from build123d import *

# Parameters (mm, degrees)
F1_DEPTH = 15.875
F2_DEPTH = 3.3528
F3_DEPTH = 5.08
F4_R     = 5.08
F5_R     = 1.27


with BuildPart() as f1:
    # F0 (on Top) → F1 (new body)
    with BuildSketch(Plane.XY):
        Polygon((0, 25.4), (0, 0), (33.02, 0), (66.04, 0), (76.2, 0), (86.36, 0), (119.38, 0), (152.4, 0), (152.4, 33.02), (152.4, 68.58), (152.4, 101.6), (127, 101.6), (76.2, 101.6), (25.4, 101.6), (0, 101.6), (0, 76.2), align=None)
        with BuildLine():
            ThreePointArc((44.0314886751, 33.02), (45.151447055, 29.2829253769), (45.5295, 25.4))
            ThreePointArc((45.5295, 25.4), (8.6879749843, 14.179260714), (33.02, 44.0314886751))
            Line((33.02, 44.0314886751), (33.02, 57.5685113249))
            ThreePointArc((33.02, 57.5685113249), (8.6879749843, 87.420739286), (45.5295, 76.2))
            ThreePointArc((45.5295, 76.2), (45.151447055, 72.3170746231), (44.0314886751, 68.58))
            Line((44.0314886751, 68.58), (57.5685113249, 68.58))
            ThreePointArc((57.5685113249, 68.58), (72.3170746231, 95.951447055), (96.3295, 76.2))
            ThreePointArc((96.3295, 76.2), (95.951447055, 72.3170746231), (94.8314886751, 68.58))
            Line((94.8314886751, 68.58), (108.3685113249, 68.58))
            ThreePointArc((108.3685113249, 68.58), (123.1170746231, 95.951447055), (147.1295, 76.2))
            ThreePointArc((147.1295, 76.2), (138.220739286, 59.4879749843), (119.38, 57.5685113249))
            Line((119.38, 57.5685113249), (119.38, 44.0314886751))
            ThreePointArc((119.38, 44.0314886751), (138.220739286, 42.1120250157), (147.1295, 25.4))
            ThreePointArc((147.1295, 25.4), (123.1170746231, 5.648552945), (108.3685113249, 33.02))
            Line((108.3685113249, 33.02), (94.8314886751, 33.02))
            ThreePointArc((94.8314886751, 33.02), (95.951447055, 29.2829253769), (96.3295, 25.4))
            ThreePointArc((96.3295, 25.4), (72.3170746231, 5.648552945), (57.5685113249, 33.02))
            Line((57.5685113249, 33.02), (44.0314886751, 33.02))
        make_face(mode=Mode.SUBTRACT)
        with BuildLine():
            ThreePointArc((45.5295, 76.2), (8.6879749843, 87.420739286), (33.02, 57.5685113249))
            ThreePointArc((33.02, 57.5685113249), (39.6337059519, 61.9662940481), (44.0314886751, 68.58))
            ThreePointArc((44.0314886751, 68.58), (45.151447055, 72.3170746231), (45.5295, 76.2))
        make_face()
        with BuildLine():
            ThreePointArc((33.02, 44.0314886751), (8.6879749843, 14.179260714), (45.5295, 25.4))
            ThreePointArc((45.5295, 25.4), (45.151447055, 29.2829253769), (44.0314886751, 33.02))
            ThreePointArc((44.0314886751, 33.02), (39.6337059519, 39.6337059519), (33.02, 44.0314886751))
        make_face()
        with BuildLine():
            ThreePointArc((66.04, 42.7773176943), (61.0000405534, 38.5968936902), (57.5685113249, 33.02))
            ThreePointArc((57.5685113249, 33.02), (72.3170746231, 5.648552945), (96.3295, 25.4))
            ThreePointArc((96.3295, 25.4), (95.951447055, 29.2829253769), (94.8314886751, 33.02))
            ThreePointArc((94.8314886751, 33.02), (91.3999594466, 38.5968936902), (86.36, 42.7773176943))
            ThreePointArc((86.36, 42.7773176943), (76.2, 45.5295), (66.04, 42.7773176943))
        make_face()
        with BuildLine():
            ThreePointArc((147.1295, 76.2), (123.1170746231, 95.951447055), (108.3685113249, 68.58))
            ThreePointArc((108.3685113249, 68.58), (112.7662940481, 61.9662940481), (119.38, 57.5685113249))
            ThreePointArc((119.38, 57.5685113249), (138.220739286, 59.4879749843), (147.1295, 76.2))
        make_face()
        with BuildLine():
            ThreePointArc((57.5685113249, 68.58), (61.0000405534, 63.0031063098), (66.04, 58.8226823057))
            ThreePointArc((66.04, 58.8226823057), (76.2, 56.0705), (86.36, 58.8226823057))
            ThreePointArc((86.36, 58.8226823057), (91.3999594466, 63.0031063098), (94.8314886751, 68.58))
            ThreePointArc((94.8314886751, 68.58), (95.951447055, 72.3170746231), (96.3295, 76.2))
            ThreePointArc((96.3295, 76.2), (72.3170746231, 95.951447055), (57.5685113249, 68.58))
        make_face()
        with BuildLine():
            ThreePointArc((119.38, 44.0314886751), (112.7662940481, 39.6337059519), (108.3685113249, 33.02))
            ThreePointArc((108.3685113249, 33.02), (123.1170746231, 5.648552945), (147.1295, 25.4))
            ThreePointArc((147.1295, 25.4), (138.220739286, 42.1120250157), (119.38, 44.0314886751))
        make_face()
        with BuildLine():
            ThreePointArc((33.02, 44.0314886751), (39.6337059519, 39.6337059519), (44.0314886751, 33.02))
            Line((44.0314886751, 33.02), (57.5685113249, 33.02))
            ThreePointArc((57.5685113249, 33.02), (61.0000405534, 38.5968936902), (66.04, 42.7773176943))
            Line((66.04, 42.7773176943), (66.04, 58.8226823057))
            ThreePointArc((66.04, 58.8226823057), (61.0000405534, 63.0031063098), (57.5685113249, 68.58))
            Line((57.5685113249, 68.58), (44.0314886751, 68.58))
            ThreePointArc((44.0314886751, 68.58), (39.6337059519, 61.9662940481), (33.02, 57.5685113249))
            Line((33.02, 57.5685113249), (33.02, 44.0314886751))
        make_face()
        with BuildLine():
            Line((86.36, 58.8226823057), (86.36, 42.7773176943))
            ThreePointArc((86.36, 42.7773176943), (91.3999594466, 38.5968936902), (94.8314886751, 33.02))
            Line((94.8314886751, 33.02), (108.3685113249, 33.02))
            ThreePointArc((108.3685113249, 33.02), (112.7662940481, 39.6337059519), (119.38, 44.0314886751))
            Line((119.38, 44.0314886751), (119.38, 57.5685113249))
            ThreePointArc((119.38, 57.5685113249), (112.7662940481, 61.9662940481), (108.3685113249, 68.58))
            Line((108.3685113249, 68.58), (94.8314886751, 68.58))
            ThreePointArc((94.8314886751, 68.58), (91.3999594466, 63.0031063098), (86.36, 58.8226823057))
        make_face()
        with BuildLine():
            Line((66.04, 58.8226823057), (66.04, 42.7773176943))
            ThreePointArc((66.04, 42.7773176943), (76.2, 45.5295), (86.36, 42.7773176943))
            Line((86.36, 42.7773176943), (86.36, 58.8226823057))
            ThreePointArc((86.36, 58.8226823057), (76.2, 56.0705), (66.04, 58.8226823057))
        make_face()
    extrude(amount=-F1_DEPTH)

    # F0 (on Top) → F2 (cut)
    with BuildSketch(Plane.XY):
        with BuildLine():
            ThreePointArc((45.5295, 76.2), (8.6879749843, 87.420739286), (33.02, 57.5685113249))
            ThreePointArc((33.02, 57.5685113249), (39.6337059519, 61.9662940481), (44.0314886751, 68.58))
            ThreePointArc((44.0314886751, 68.58), (45.151447055, 72.3170746231), (45.5295, 76.2))
        make_face()
        with BuildLine():
            ThreePointArc((33.02, 44.0314886751), (8.6879749843, 14.179260714), (45.5295, 25.4))
            ThreePointArc((45.5295, 25.4), (45.151447055, 29.2829253769), (44.0314886751, 33.02))
            ThreePointArc((44.0314886751, 33.02), (39.6337059519, 39.6337059519), (33.02, 44.0314886751))
        make_face()
        with BuildLine():
            ThreePointArc((66.04, 42.7773176943), (61.0000405534, 38.5968936902), (57.5685113249, 33.02))
            ThreePointArc((57.5685113249, 33.02), (72.3170746231, 5.648552945), (96.3295, 25.4))
            ThreePointArc((96.3295, 25.4), (95.951447055, 29.2829253769), (94.8314886751, 33.02))
            ThreePointArc((94.8314886751, 33.02), (91.3999594466, 38.5968936902), (86.36, 42.7773176943))
            ThreePointArc((86.36, 42.7773176943), (76.2, 45.5295), (66.04, 42.7773176943))
        make_face()
        with BuildLine():
            ThreePointArc((57.5685113249, 68.58), (61.0000405534, 63.0031063098), (66.04, 58.8226823057))
            ThreePointArc((66.04, 58.8226823057), (76.2, 56.0705), (86.36, 58.8226823057))
            ThreePointArc((86.36, 58.8226823057), (91.3999594466, 63.0031063098), (94.8314886751, 68.58))
            ThreePointArc((94.8314886751, 68.58), (95.951447055, 72.3170746231), (96.3295, 76.2))
            ThreePointArc((96.3295, 76.2), (72.3170746231, 95.951447055), (57.5685113249, 68.58))
        make_face()
        with BuildLine():
            ThreePointArc((147.1295, 76.2), (123.1170746231, 95.951447055), (108.3685113249, 68.58))
            ThreePointArc((108.3685113249, 68.58), (112.7662940481, 61.9662940481), (119.38, 57.5685113249))
            ThreePointArc((119.38, 57.5685113249), (138.220739286, 59.4879749843), (147.1295, 76.2))
        make_face()
        with BuildLine():
            ThreePointArc((119.38, 44.0314886751), (112.7662940481, 39.6337059519), (108.3685113249, 33.02))
            ThreePointArc((108.3685113249, 33.02), (123.1170746231, 5.648552945), (147.1295, 25.4))
            ThreePointArc((147.1295, 25.4), (138.220739286, 42.1120250157), (119.38, 44.0314886751))
        make_face()
    extrude(amount=-F2_DEPTH, mode=Mode.SUBTRACT)

    # F0 (on Top) → F3 (cut)
    with BuildSketch(Plane.XY):
        with BuildLine():
            ThreePointArc((33.02, 44.0314886751), (39.6337059519, 39.6337059519), (44.0314886751, 33.02))
            Line((44.0314886751, 33.02), (57.5685113249, 33.02))
            ThreePointArc((57.5685113249, 33.02), (61.0000405534, 38.5968936902), (66.04, 42.7773176943))
            Line((66.04, 42.7773176943), (66.04, 58.8226823057))
            ThreePointArc((66.04, 58.8226823057), (61.0000405534, 63.0031063098), (57.5685113249, 68.58))
            Line((57.5685113249, 68.58), (44.0314886751, 68.58))
            ThreePointArc((44.0314886751, 68.58), (39.6337059519, 61.9662940481), (33.02, 57.5685113249))
            Line((33.02, 57.5685113249), (33.02, 44.0314886751))
        make_face()
        with BuildLine():
            Line((86.36, 58.8226823057), (86.36, 42.7773176943))
            ThreePointArc((86.36, 42.7773176943), (91.3999594466, 38.5968936902), (94.8314886751, 33.02))
            Line((94.8314886751, 33.02), (108.3685113249, 33.02))
            ThreePointArc((108.3685113249, 33.02), (112.7662940481, 39.6337059519), (119.38, 44.0314886751))
            Line((119.38, 44.0314886751), (119.38, 57.5685113249))
            ThreePointArc((119.38, 57.5685113249), (112.7662940481, 61.9662940481), (108.3685113249, 68.58))
            Line((108.3685113249, 68.58), (94.8314886751, 68.58))
            ThreePointArc((94.8314886751, 68.58), (91.3999594466, 63.0031063098), (86.36, 58.8226823057))
        make_face()
    extrude(amount=-F3_DEPTH, mode=Mode.SUBTRACT)

    # F4
    f4_edges = [f1.edges().sort_by_distance(p)[0] for p in [
        (0, 0, -7.9375),
        (152.4, 0, -7.9375),
        (152.4, 101.6, -7.9375),
        (0, 101.6, -7.9375),
    ]]
    fillet(f4_edges, radius=F4_R)

    # F5
    f5_edges = [f1.edges().sort_by_distance(p)[0] for p in [
        (86.36, 58.822682, -1.6764),
        (94.831489, 68.58, -1.6764),
        (108.368511, 68.58, -1.6764),
        (119.38, 57.568511, -1.6764),
        (119.38, 44.031489, -1.6764),
        (108.368511, 33.02, -1.6764),
        (94.831489, 33.02, -1.6764),
        (86.36, 42.777318, -1.6764),
        (66.04, 42.777318, -1.6764),
        (57.568511, 33.02, -1.6764),
        (44.031489, 33.02, -1.6764),
        (33.02, 44.031489, -1.6764),
        (33.02, 57.568511, -1.6764),
        (44.031489, 68.58, -1.6764),
        (57.568511, 68.58, -1.6764),
        (66.04, 58.822682, -1.6764),
    ]]
    fillet(f5_edges, radius=F5_R)


solid = f1.part
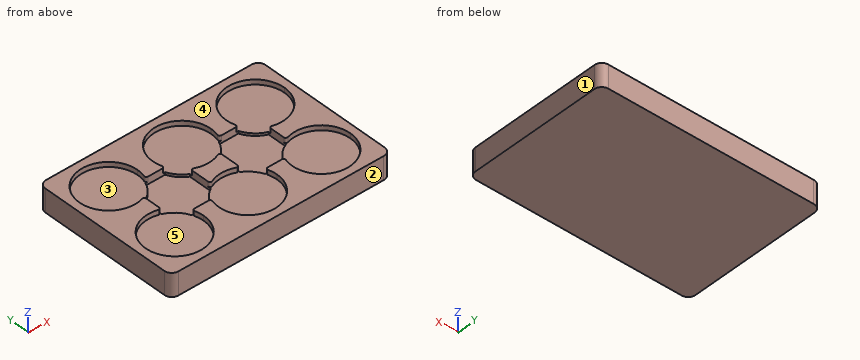
Model file for the job. Use its own axes, mm. Face numbers are marked on the shaded views. A direction names the side the tool comes from. Coordinates: 2 decimals unless noted, no trailing zeros. Loops run counter-clockwise (first coordinate to the right, second up) from the corner with the lowest first, then second, coordinate; pieces in that order, holes last. Notation, with made-up numbers: (41.5, 52) -> (49.5, 52) arc R23 cw to (49.5, 82) -> close; hole circle Ø8 at (88, 65). An arc over 180 degrees is marked (long way). Use one line per item in the form item = value. Start each with the question number.
(1) Cut at A-A on x = 127. Give the cut face in (y, z) (1 decimal), and give its area (3 significant figures).
(2) Cut at D-D on y = 65. Give the cut face in (x, z) (3 decimals).
(3) Probe probe 1 along Y at (x, z) = (76.2, -1.9); probe 2 along X at (y, z) = (25.4, -2); probe 3 along Y at (x, z) = (83, -3). List the from-to ranges inside material, lowest first. Write a range as from..to.
(4) Cut at B-B on y = 87. Give the cut face in (x, z) (3 decimals).
(5) Cut at C-C on x = 88. Give the cut face in (y, z) (3 decimals).
(6) Pull direction X, two halves, no side cores. Call the marked faces 1, 2 and 3: pulls with the +X half, pulls with the -X half, needs draft (parallel to the pull), parting line crosses it, or undercut.
(7) Tool access for the marked faces 4 and 5: list every direction of +Z, -Z, +X, -X, +Y, -Y with a clear straight run to the whole face (end or side of a thin tool).
(8) Flat gauge pin, fed straight in: pin 1 (2 mm diameter, centred on x = 133.5, y = 78.5, fed in from +Z). Where does the tip first touch, or does it go through?
Values:
q1.outline = (0, -15.9) -> (101.6, -15.9) -> (101.6, 0) -> (96.3, 0) -> (96.3, -3.4) -> (56.1, -3.4) -> (56.1, 0) -> (45.5, 0) -> (45.5, -3.4) -> (5.3, -3.4) -> (5.3, 0) -> (0, 0) -> close
q1.area = 1,340 mm2
q2.outline = (0, -15.875) -> (152.4, -15.875) -> (152.4, 0) -> (143.726, 0) -> (143.726, -3.353) -> (110.274, -3.353) -> (110.274, -5.08) -> (92.926, -5.08) -> (92.926, -3.353) -> (59.474, -3.353) -> (59.474, -5.08) -> (42.126, -5.08) -> (42.126, -3.353) -> (8.674, -3.353) -> (8.674, 0) -> (0, 0) -> close
q3.probe_1 = 0..5.27, 45.53..56.07, 96.33..101.6
q3.probe_2 = 0..5.27, 45.53..56.07, 96.33..106.87, 147.13..152.4
q3.probe_3 = 0..6.45, 44.35..57.25, 95.15..101.6
q4.outline = (0, -15.875) -> (152.4, -15.875) -> (152.4, 0) -> (143.987, 0) -> (143.987, -3.353) -> (110.013, -3.353) -> (110.013, 0) -> (93.187, 0) -> (93.187, -3.353) -> (59.213, -3.353) -> (59.213, 0) -> (42.387, 0) -> (42.387, -3.353) -> (8.413, -3.353) -> (8.413, 0) -> (0, 0) -> close
q5.outline = (0, -15.875) -> (101.6, -15.875) -> (101.6, 0) -> (92.508, 0) -> (92.508, -3.353) -> (59.892, -3.353) -> (59.892, -5.08) -> (41.708, -5.08) -> (41.708, -3.353) -> (9.092, -3.353) -> (9.092, 0) -> (0, 0) -> close
q6.face_1 = pulls with the +X half
q6.face_2 = needs draft
q6.face_3 = undercut
q7.face_4 = +Z, +X, -X, +Y, -Y
q7.face_5 = +Z
q8.pin_1 = -3.35
